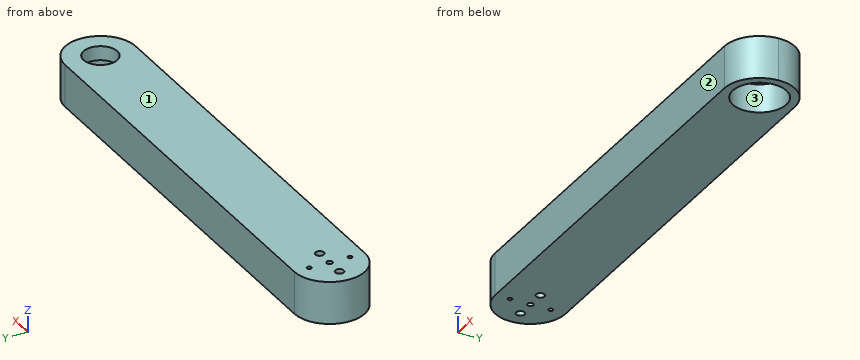
```python
from build123d import *

# Parameters (mm, degrees)
EXTRUDE_1_DEPTH          = 15
CUT_EXTRUDE_3_DEPTH      = 90.652105385
CUT_EXTRUDE_3_DEPTH_BACK = 90.652105385
SKETCH_7_R               = 1.5
SKETCH_8_R               = 9.5
CUT_EXTRUDE_4_DEPTH      = 10
SKETCH_9_R               = 6
CUT_EXTRUDE_10_DEPTH     = 20
M2X0_4_1_D               = 1.6
M2X0_4_2_D               = 1.6


with BuildPart() as part:
    # ｽｹｯﾁ2 → ﾎﾞｽ - 押し出し1 (new body)
    with BuildSketch(Plane.XY):
        with BuildLine():
            ThreePointArc((-62.5, 0), (-66.161165235, 8.838834765), (-75, 12.5))
            Line((-75, 12.5), (-75, 1.05))
            ThreePointArc((-75, 1.05), (-74.25753788, 0.74246212), (-73.95, 0))
            ThreePointArc((-73.95, 0), (-74.25753788, -0.74246212), (-75, -1.05))
            Line((-75, -1.05), (-75, -12.5))
            ThreePointArc((-75, -12.5), (-66.161165235, -8.838834765), (-62.5, 0))
        make_face()
        with BuildLine():
            Line((-75, 1.05), (-75, 12.5))
            ThreePointArc((-75, 12.5), (-87.5, 0), (-75, -12.5))
            Line((-75, -12.5), (-75, -1.05))
            ThreePointArc((-75, -1.05), (-76.05, 0), (-75, 1.05))
        make_face()
        with BuildLine():
            Line((75, 12.5), (-75, 12.5))
            ThreePointArc((-75, 12.5), (-66.161165235, 8.838834765), (-62.5, 0))
            ThreePointArc((-62.5, 0), (-66.161165235, -8.838834765), (-75, -12.5))
            Line((-75, -12.5), (75, -12.5))
            ThreePointArc((75, -12.5), (62.5, 0), (75, 12.5))
        make_face()
        with BuildLine():
            ThreePointArc((87.5, 0), (83.838834765, 8.838834765), (75, 12.5))
            Line((75, 12.5), (75, 1.05))
            ThreePointArc((75, 1.05), (75.74246212, 0.74246212), (76.05, 0))
            ThreePointArc((76.05, 0), (75.74246212, -0.74246212), (75, -1.05))
            Line((75, -1.05), (75, -12.5))
            ThreePointArc((75, -12.5), (83.838834765, -8.838834765), (87.5, 0))
        make_face()
        with BuildLine():
            Line((75, 1.05), (75, 12.5))
            ThreePointArc((75, 12.5), (62.5, 0), (75, -12.5))
            Line((75, -12.5), (75, -1.05))
            ThreePointArc((75, -1.05), (73.95, 0), (75, 1.05))
        make_face()
    extrude(amount=EXTRUDE_1_DEPTH)

    # ｽｹｯﾁ7 → ｶｯﾄ - 押し出し3 (cut, two sides: drawn at the far end of the back side and taken through both)
    with BuildSketch(Plane.XY.offset(-CUT_EXTRUDE_3_DEPTH_BACK)):
        with Locations((-68.5, 0)):
            Circle(SKETCH_7_R)
        with Locations((-81.5, 0)):
            Circle(SKETCH_7_R)
    extrude(amount=CUT_EXTRUDE_3_DEPTH + CUT_EXTRUDE_3_DEPTH_BACK, mode=Mode.SUBTRACT)

    # ｽｹｯﾁ8 → ｶｯﾄ - 押し出し4 (cut)
    with BuildSketch(Plane.XY):
        with Locations((75, 0)):
            Circle(SKETCH_8_R)
    extrude(amount=CUT_EXTRUDE_4_DEPTH, mode=Mode.SUBTRACT)

    # ｽｹｯﾁ9 → ｶｯﾄ - 押し出し10 (cut)
    with BuildSketch(Plane.XY):
        with Locations((75, 0)):
            Circle(SKETCH_9_R)
    extrude(amount=CUT_EXTRUDE_10_DEPTH, mode=Mode.SUBTRACT)

    # M2x0.4 ねじ穴1 (through all)
    with Locations(Plane.XY.offset(15)):
        with Locations((-75, 7.2), (-67.8, 0), (-75, -7.2)):
            Hole(M2X0_4_1_D / 2)

    # M2x0.4 ねじ穴2 (through all)
    with Locations(Plane.XY.offset(15)):
        with Locations((-67.8, 0)):
            Hole(M2X0_4_2_D / 2)


solid = part.part
```
Work out the finished part from the listing and answer in its coordinate system (mm). Face numbers are marked on the shaded views. Give positions to 0.01 mm unless a question says otherwise; leave off trailing zeros. Loops run counter-clockwise (first coordinate to the right, second up) from the corner with the lowest first, then second, coordinate; pieces in that order, holes last. Notation, with made-up numbers: (16.25, 60) -> (36.25, 60) arc R12 cw to (36.25, 71) -> close; hole circle Ø7 at (52.5, 31). An arc over 180 degrees is marked (long way). Write item = value, one per line. Start each with the question number.
(1) Find section A-A on z = 3.75. Give the vertices of the cut face in (x, y).
(2) Find section C-C on y = 4.25. Give the vertices of the cut face in (x, z), and give its area (3 significant figures).
(3) Given pin 1 Ø2.5 at (x, y) = (-81.5, 0) entering from +Z; pin 2 Ø6 at (y, z) = (-7, 12) entering from -X; pin 3 Ø8 at (y, z) = (-7, 10) entering from +X; pin 4 Ø1 at (y, z) = (9.5, 5.5) entering from +X, each flat-ended and moving along its own axis, determine where each tip first touches the part or whether it passes through.
(4) The mould has two halves that part along Y. Classify the marked faces 1, 2 and 3: +Y half, -Y half, draft (parallel to the pull), parting line (faces both ways), or undercut.
(5) Find the intervals of material crossed by probe 1 along Y at (x, z) = (75, 12.3); probe 2 along Y at (x, z) = (-68.5, 6.5); probe 3 along X at (y, z) = (-6.75, 1), in increasing order. Write a range as from..to.
(6) Find section D-D on z = 12. Give the vertices of the cut face in (x, y).
(7) Find section B-B on x = 72.5. Give the vertices of the cut face in (y, z), and give its area (3 significant figures).
From the geometry:
q1.outline = (-75, -12.5) -> (75, -12.5) arc R12.5 ccw to (75, 12.5) -> (-75, 12.5) arc R12.5 ccw to start; hole circle Ø3 at (-81.5, 0); hole circle Ø2.1 at (-75, 0); hole circle Ø1.6 at (-75, -7.2); hole circle Ø1.6 at (-75, 7.2); hole circle Ø3 at (-68.5, 0); hole circle Ø19 at (75, 0)
q2.outline = (-86.76, 0) -> (66.5, 0) -> (66.5, 10) -> (70.76, 10) -> (70.76, 15) -> (-86.76, 15) -> close; (79.24, 10) -> (83.5, 10) -> (83.5, 0) -> (86.76, 0) -> (86.76, 15) -> (79.24, 15) -> close
q2.area = 2,390 mm^2
q3.pin_1 = through
q3.pin_2 = -86.84
q3.pin_3 = 87.13
q3.pin_4 = 83.67
q4.face_1 = draft
q4.face_2 = -Y half
q4.face_3 = undercut
q5.probe_1 = -12.5..-6, 6..12.5
q5.probe_2 = -12.5..-1.5, 1.5..12.5
q5.probe_3 = -85.52..-75.66, -74.34..68.32, 81.68..85.52
q6.outline = (-75, -12.5) -> (75, -12.5) arc R12.5 ccw to (75, 12.5) -> (-75, 12.5) arc R12.5 ccw to start; hole circle Ø3 at (-81.5, 0); hole circle Ø2.1 at (-75, 0); hole circle Ø1.6 at (-75, -7.2); hole circle Ø1.6 at (-75, 7.2); hole circle Ø3 at (-68.5, 0); hole circle Ø12 at (75, 0)
q7.outline = (-12.5, 0) -> (-9.17, 0) -> (-9.17, 10) -> (-5.45, 10) -> (-5.45, 15) -> (-12.5, 15) -> close; (5.45, 10) -> (9.17, 10) -> (9.17, 0) -> (12.5, 0) -> (12.5, 15) -> (5.45, 15) -> close
q7.area = 137 mm^2
